The model under review builds one solid part; all positions refer to its coordinate system, in mm. A direction names the side the tool comes from. Give positions to 0.01 mm unless a question says otherwise; leave off trailing zeros. Use CSV: the item, a comma, the result in double quotes. Start each with the question number.
```python
from build123d import *

# Parameters (mm, degrees)
F1_DEPTH = 40
F3_DEPTH = 40
F5_DEPTH = 20


with BuildPart() as f1:
    # F0 (on Front) → F1 (new body)
    with BuildSketch(Plane.XZ):
        Polygon((165, 165), (165, 225), (-165, 225), (-165, 165), (-225, 165), (-225, -165), (-165, -165), (-165, -225), (165, -225), (165, -165), (225, -165), (225, 165), align=None)
    extrude(amount=F1_DEPTH)

    # F2 (on face) → F3 (join, through all)
    with BuildSketch(Plane.XZ.offset(40)):
        with BuildLine():
            Line((-201, 171), (-201, 165))
            Line((-201, 165), (-189, 165))
            Line((-189, 165), (-189, 171))
            Line((-189, 171), (-185, 171))
            Line((-185, 171), (-185, 181))
            ThreePointArc((-185, 181), (-195, 183.6794919243), (-205, 181))
            Line((-205, 181), (-205, 171))
            Line((-205, 171), (-201, 171))
        make_face()
        with BuildLine():
            Line((-171, 189), (-165, 189))
            Line((-165, 189), (-165, 201))
            Line((-165, 201), (-171, 201))
            Line((-171, 201), (-171, 205))
            Line((-171, 205), (-181, 205))
            ThreePointArc((-181, 205), (-183.6794919243, 195), (-181, 185))
            Line((-181, 185), (-171, 185))
            Line((-171, 185), (-171, 189))
        make_face()
        with BuildLine():
            Line((171, 201), (165, 201))
            Line((165, 201), (165, 189))
            Line((165, 189), (171, 189))
            Line((171, 189), (171, 185))
            Line((171, 185), (181, 185))
            ThreePointArc((181, 185), (183.6794919243, 195), (181, 205))
            Line((181, 205), (171, 205))
            Line((171, 205), (171, 201))
        make_face()
        with BuildLine():
            Line((189, 171), (189, 165))
            Line((189, 165), (201, 165))
            Line((201, 165), (201, 171))
            Line((201, 171), (205, 171))
            Line((205, 171), (205, 181))
            ThreePointArc((205, 181), (195, 183.6794919243), (185, 181))
            Line((185, 181), (185, 171))
            Line((185, 171), (189, 171))
        make_face()
        with BuildLine():
            Line((201, -165), (189, -165))
            Line((189, -165), (189, -171))
            Line((189, -171), (185, -171))
            Line((185, -171), (185, -181))
            ThreePointArc((185, -181), (195, -183.6794919243), (205, -181))
            Line((205, -181), (205, -171))
            Line((205, -171), (201, -171))
            Line((201, -171), (201, -165))
        make_face()
        with BuildLine():
            Line((165, -189), (165, -201))
            Line((165, -201), (171, -201))
            Line((171, -201), (171, -205))
            Line((171, -205), (181, -205))
            ThreePointArc((181, -205), (183.6794919243, -195), (181, -185))
            Line((181, -185), (171, -185))
            Line((171, -185), (171, -189))
            Line((171, -189), (165, -189))
        make_face()
        with BuildLine():
            Line((-165, -201), (-165, -189))
            Line((-165, -189), (-171, -189))
            Line((-171, -189), (-171, -185))
            Line((-171, -185), (-181, -185))
            ThreePointArc((-181, -185), (-183.6794919243, -195), (-181, -205))
            Line((-181, -205), (-171, -205))
            Line((-171, -205), (-171, -201))
            Line((-171, -201), (-165, -201))
        make_face()
        with BuildLine():
            Line((-189, -165), (-201, -165))
            Line((-201, -165), (-201, -171))
            Line((-201, -171), (-205, -171))
            Line((-205, -171), (-205, -181))
            ThreePointArc((-205, -181), (-195, -183.6794919243), (-185, -181))
            Line((-185, -181), (-185, -171))
            Line((-185, -171), (-189, -171))
            Line((-189, -171), (-189, -165))
        make_face()
    extrude(amount=-F3_DEPTH)

    # F4 (on face) → F5 (join)
    with BuildSketch(Plane(origin=(0, 0, 0), x_dir=(-1, 0, 0), z_dir=(0, 1, 0))):
        Polygon((165, 201), (165, 225), (-165, 225), (-165, 201), (-165, 189), (-165, 165), (-189, 165), (-201, 165), (-225, 165), (-225, -165), (-201, -165), (-189, -165), (-165, -165), (-165, -189), (-165, -201), (-165, -225), (165, -225), (165, -201), (165, -189), (165, -165), (189, -165), (201, -165), (225, -165), (225, 165), (201, 165), (189, 165), (165, 165), (165, 189), align=None)
        with BuildLine():
            Line((225, -225), (225, -165))
            Line((225, -165), (201, -165))
            Line((201, -165), (201, -171))
            Line((201, -171), (205, -171))
            Line((205, -171), (205, -181))
            ThreePointArc((205, -181), (195, -183.6794919243), (185, -181))
            Line((185, -181), (185, -171))
            Line((185, -171), (189, -171))
            Line((189, -171), (189, -165))
            Line((189, -165), (165, -165))
            Line((165, -165), (165, -189))
            Line((165, -189), (171, -189))
            Line((171, -189), (171, -185))
            Line((171, -185), (181, -185))
            ThreePointArc((181, -185), (183.6794919243, -195), (181, -205))
            Line((181, -205), (171, -205))
            Line((171, -205), (171, -201))
            Line((171, -201), (165, -201))
            Line((165, -201), (165, -225))
            Line((165, -225), (225, -225))
        make_face()
        with BuildLine():
            Line((-201, -165), (-225, -165))
            Line((-225, -165), (-225, -225))
            Line((-225, -225), (-165, -225))
            Line((-165, -225), (-165, -201))
            Line((-165, -201), (-171, -201))
            Line((-171, -201), (-171, -205))
            Line((-171, -205), (-181, -205))
            ThreePointArc((-181, -205), (-183.6794919243, -195), (-181, -185))
            Line((-181, -185), (-171, -185))
            Line((-171, -185), (-171, -189))
            Line((-171, -189), (-165, -189))
            Line((-165, -189), (-165, -165))
            Line((-165, -165), (-189, -165))
            Line((-189, -165), (-189, -171))
            Line((-189, -171), (-185, -171))
            Line((-185, -171), (-185, -181))
            ThreePointArc((-185, -181), (-195, -183.6794919243), (-205, -181))
            Line((-205, -181), (-205, -171))
            Line((-205, -171), (-201, -171))
            Line((-201, -171), (-201, -165))
        make_face()
        with BuildLine():
            Line((-165, 201), (-165, 225))
            Line((-165, 225), (-225, 225))
            Line((-225, 225), (-225, 165))
            Line((-225, 165), (-201, 165))
            Line((-201, 165), (-201, 171))
            Line((-201, 171), (-205, 171))
            Line((-205, 171), (-205, 181))
            ThreePointArc((-205, 181), (-195, 183.6794919243), (-185, 181))
            Line((-185, 181), (-185, 171))
            Line((-185, 171), (-189, 171))
            Line((-189, 171), (-189, 165))
            Line((-189, 165), (-165, 165))
            Line((-165, 165), (-165, 189))
            Line((-165, 189), (-171, 189))
            Line((-171, 189), (-171, 185))
            Line((-171, 185), (-181, 185))
            ThreePointArc((-181, 185), (-183.6794919243, 195), (-181, 205))
            Line((-181, 205), (-171, 205))
            Line((-171, 205), (-171, 201))
            Line((-171, 201), (-165, 201))
        make_face()
        with BuildLine():
            Line((225, 165), (225, 225))
            Line((225, 225), (165, 225))
            Line((165, 225), (165, 201))
            Line((165, 201), (171, 201))
            Line((171, 201), (171, 205))
            Line((171, 205), (181, 205))
            ThreePointArc((181, 205), (183.6794919243, 195), (181, 185))
            Line((181, 185), (171, 185))
            Line((171, 185), (171, 189))
            Line((171, 189), (165, 189))
            Line((165, 189), (165, 165))
            Line((165, 165), (189, 165))
            Line((189, 165), (189, 171))
            Line((189, 171), (185, 171))
            Line((185, 171), (185, 181))
            ThreePointArc((185, 181), (195, 183.6794919243), (205, 181))
            Line((205, 181), (205, 171))
            Line((205, 171), (201, 171))
            Line((201, 171), (201, 165))
            Line((201, 165), (225, 165))
        make_face()
    extrude(amount=-F5_DEPTH)


solid = f1.part
```
1. Mouldability with a two-part tool opening along Z and no side actions: class faces 6 (the face through (177, -30, -165)), 7 (the face through (-185, -30, -176)), 8 (the face through (195, -20, -195)), 9 (the face through (195.15, -30.14, 183.68)) as pulls with the +Z half, pulls with the -Z half, needs draft (parallel to the pull), parting line crosses it, or undercut.
2. Clearance check with flat-ended pins moving along their axes: pin 1 (10 mm diameter, centred on x = 213, y = -26, fed in from -Z); pin 2 (16 mm diameter, centred on x = -218, y = -32.5, fed in from +Z); pin 3 (2 mm diameter, centred on y = -29.5, z = 187, fed in from -X). State where each tip first meets the part, or that it passes through.
3. Tool access review of faces 1 (the face through (-177, -30, 165)), 2 (the face through (176, -30, -205)), 3 (the face through (165, -30, 213)), 4 (the face through (213, -30, -165)), 5 (the face through (-176, -30, 185)): name each direction out of +Z, -Z, +X, -X, +Y, -Y from which nothing blocks a thin tool from reaching the whole face with its end or side.
4. To check wall thickness, follow L1, parallel to Z at x = 187, y = -36; L2, parallel to Z at x = -188, y = -33; L3, parallel to X at y = -23.5, z = 191. State the ranges of each line that lie inside material, in increasing order. Write a range as [from, to].
Answers follow:
1,face 6,"undercut"
1,face 7,"needs draft"
1,face 8,"undercut"
1,face 9,"pulls with the +Z half"
2,pin 1,"stops at z = -165"
2,pin 2,"stops at z = 165"
2,pin 3,"stops at x = -182.41"
3,face 1,"-Y"
3,face 2,"-Z, +X, -Y"
3,face 3,"+Z, -Y"
3,face 4,"+X, -Y"
3,face 5,"-X, -Y"
4,L1,"z = [-182.01, -171], [-165, 165], [171, 182.01]"
4,L2,"z = [-182.41, -171], [-165, 165], [171, 182.41]"
4,L3,"x = [-183.28, 183.28]"
